Design review of the part built by this model. Coordinates are the model's own, in mm. Face numbers are marked on the shaded views. A direction names the side the tool comes from. Coordinates: 2 decimals unless noted, no trailing zeros. Loops run counter-clockwise (first coordinate to the right, second up) from the corner with the lowest first, then second, coordinate; pieces in that order, holes last.
Q1. Add section C-C on y = 0. Give the boundary of the cut face in (x, z).
Q2. Add section B-B on x = 0.75. Give the boundary of the cut face in (y, z).
Q3. For P1, Ø5, axis at x = -1.5, y = 0.5, coming from the +Z side; P2, Ø3.5, axis at x = -1, y = -0.5, coming from the -Z side; P3, Ø5, axis at x = 0.5, y = -9, coming from the +Z side, all flat-tipped, find the tip position at first contact; note any pin that passes through.
Q4. Machinability: for the marked faces 1 and 2, which of the approach directions +Z, -Z, +X, -X, +Y, -Y give a long, thin tool a straight path to every point of the face, cutting with its end or side? Answer none if there is none.
Q5. Draft analysis for pull direction Y (two halves, no side actions). For the marked faces 3, 4 and 5, state which applies: released by +Y, released by -Y, zero draft, split by the parting line, or undercut.
Q6. Add section D-D on x = -7. Give the boundary of the cut face in (y, z), and give its area (3 significant figures).
Q7. Add section A-A on z = 0. Give the boundary of the cut face in (x, y), and give its area (3 significant figures).
Q8. Wall thickness on probe 1 along X at (y, z) = (-8, 0.5); probe 2 along Y at (x, z) = (-6.75, 0); probe 3 along Y at (x, z) = (1, 9): over which ranges is each line inside the solid? List them lowest first.
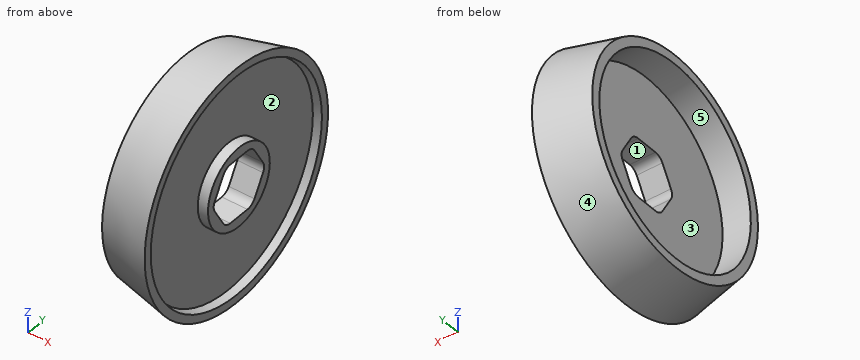
Autodesk Inventor part; units mm, degrees
ref_plane "YZ Plane" through (0, 0, 0) normal (1, 0, 0) x (0, 1, 0)
ref_plane "XZ Plane" through (0, 0, 0) normal (0, 1, 0) x (-1, 0, 0)
ref_plane "XY Plane" through (0, 0, 0) normal (0, 0, 1) x (1, 0, 0)
sketch "Sketch1" plane through (0, 0, 0) normal (0, 1, 0) x (-1, 0, 0)
  line L0 (0, 0) -> (3, 0) construction
  line L1 (3, 0) -> (3, -5.75) construction
  line L2 (3, -5.75) -> (0, -5.75) construction
  line L3 (0, -5.75) -> (0, 0) construction
  line L4 (0, -5.75) -> (3, -5.75)
  line L5 (3, -5.75) -> (3, -25)
  line L6 (3, -25) -> (0, -25)
  line L7 (0, -25) -> (0, -5.75)
  line L8 (8.5, -25) -> (-1.5, -25) construction
  line L9 (-1.5, -25) -> (-1.5, -19)
  line L10 (-1.5, -19) -> (8.5, -19)
  line L11 (8.5, -19) -> (8.5, -25)
  line L12 (-1.5, -23) -> (8.5, -20.7831)
  line L13 (-1.5, -21.4636) -> (8.5, -19.2466)
  line L14 (3, -5.75) -> (5, -5.75)
  line L15 (5, -5.75) -> (5, -9.75)
  line L16 (5, -9.75) -> (3, -9.75)
  line L17 (3, -9.75) -> (3, -5.75)
  line L18 (0, -5.75) -> (-2, -5.75)
  line L19 (-2, -5.75) -> (-2, -7.75)
  line L20 (-2, -7.75) -> (0, -7.75)
  line L21 (0, -7.75) -> (0, -5.75)
  point P0 (3, -19)
  point P1 (0, -19)
  point P2 (0, -21.131)
  point P3 (3, -20.466)
  point P4 (3, -9.75)
  point P5 (0, -7.75)
  dimension "d21" = 3
  dimension "d22" = 5.75
  dimension "d24" = 1.5
  dimension "d25" = 10
  dimension "d26" = 6
  dimension "d27" = 2
  dimension "d29" = 23
  dimension "d30" = 1.5
  dimension "d34" = 2
  dimension "d35" = 4
  dimension "d36" = 2
  dimension "d37" = 2
  dimension "d38" = 12.5
revolve "Revolution1" add sketch "Sketch1" angle 360 about axis through (0, 0, 0) along (-1, 0, 0) contours L4 L5 L10 L7 | L7 L20 L19 L18 | L10 L5 L13 L7 | L10 L11 L13 L5 | L13 L5 L12 L7 | L7 L12 L9 L13 | L13 L11 L12 L5
sketch "Sketch5" plane through (-3, 0, 0) normal (-1, 0, 0) x (0, 0, 1)
  line L0 (0, 0) -> (-5.75, 0) construction
  line L1 (-5.75, 3.3198) -> (0, 6.6395)
  line L2 (0, 6.6395) -> (5.75, 3.3198)
  line L3 (5.75, 3.3198) -> (5.75, -3.3198)
  line L4 (5.75, -3.3198) -> (0, -6.6395)
  line L5 (0, -6.6395) -> (-5.75, -3.3198)
  line L6 (-5.75, -3.3198) -> (-5.75, 3.3198)
  circle A0 centre (0, 0) radius 5.75
  circle A1 centre (0, 0) radius 19
  circle A2 centre (0, 0) radius 5.75
extrude "Extrusion4" cut sketch "Sketch5" along normal through all both and the other way through all contours L1 A0 L6 | L1 L2 A0 | A0 | A0 L5 L6 | L2 L3 A0 | A0 L4 L5 | L3 L4 A0
fillet "Fillet4" radius 2 6 edges at (-0.5, -3.3198, -5.75) (-0.5, 3.3198, -5.75) (-0.5, 6.6395, 0) (-0.5, -6.6395, 0) (-0.5, -3.3198, 5.75) (-0.5, 3.3198, 5.75)
properties part number "Clutch" material "Stainless Steel"
Entries:
1. outline: (-8.5, -20.78) - (1.5, -23) - (1.5, -21.46) - (0, -21.13) - (0, -7.75) - (2, -7.75) - (2, -5.75) - (-3, -5.75) - (-3, -19) - (-8.5, -19) - close; (-8.5, 19) - (-3, 19) - (-3, 5.75) - (2, 5.75) - (2, 7.75) - (0, 7.75) - (0, 21.13) - (1.5, 21.46) - (1.5, 23) - (-8.5, 20.78) - close
2. outline: circle Ø45.67 at (0, 0); circle Ø15.5 at (0, 0); hole circle Ø42.59 at (0, 0); hole (-6.06, -1) - (-3.9, -4.75) arc R2 ccw to (-2.17, -5.75) - (2.17, -5.75) arc R2 ccw to (3.9, -4.75) - (6.06, -1) arc R2 ccw to (6.06, 1) - (3.9, 4.75) arc R2 ccw to (2.17, 5.75) - (-2.17, 5.75) arc R2 ccw to (-3.9, 4.75) - (-6.06, 1) arc R2 ccw to start
3. P1: stops at z = 22.89
3. P2: stops at z = -22.83
3. P3: stops at z = 22
4. face 1: +X, -X
4. face 2: +X
5. face 3: undercut
5. face 4: split by the parting line
5. face 5: undercut
6. outline: circle Ø42.23 at (0, 0); hole circle Ø38 at (0, 0)
6. area: 267 mm2
7. outline: (-8.5, -20.78) - (1.5, -23) - (1.5, -21.46) - (0, -21.13) - (0, -7.75) - (2, -7.75) - (2, -6.33) - (-3, -6.33) - (-3, -19) - (-8.5, -19) - close; (-8.5, 19) - (-3, 19) - (-3, 6.33) - (2, 6.33) - (2, 7.75) - (0, 7.75) - (0, 21.13) - (1.5, 21.46) - (1.5, 23) - (-8.5, 20.78) - close
7. area: 133 mm2
8. probe 1: x = -3 to 0
8. probe 2: y = -21.17 to -19, 19 to 21.17
8. probe 3: y = -21.05 to -19.36, 19.36 to 21.05
